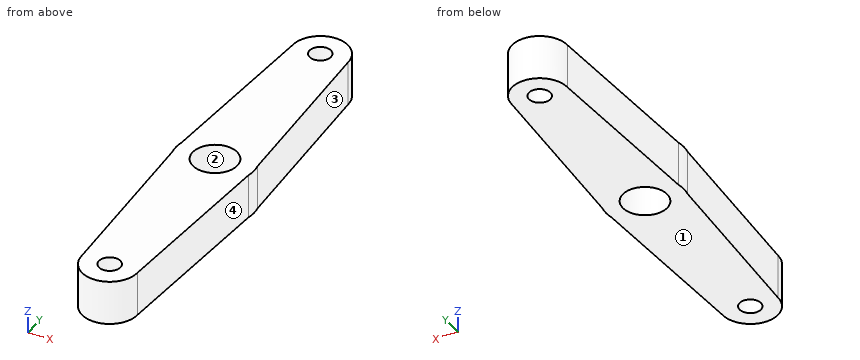
from build123d import *

# Parameters (mm, degrees)
SKETCH001_R   = 2
SKETCH001_R_2 = 0.965047
PAD_DEPTH     = 4


with BuildPart() as part:
    # Sketch001 → Pad (new body)
    with BuildSketch(Plane.XY):
        with BuildLine():
            ThreePointArc((-3.420895, 0.739919), (-3.5, 0), (-3.420895, -0.739919))
            Line((-2.5, -17), (-3.420895, -0.739919))
            ThreePointArc((-2.5, -17), (0, -19.5), (2.5, -17))
            Line((2.5, -17), (3.420895, -0.739919))
            ThreePointArc((3.420895, -0.739919), (3.5, 0), (3.420895, 0.739919))
            Line((3.420895, 0.739919), (2.5, 17))
            ThreePointArc((2.5, 17), (0, 19.5), (-2.5, 17))
            Line((-3.420895, 0.739919), (-2.5, 17))
        make_face()
        Circle(SKETCH001_R, mode=Mode.SUBTRACT)
        with Locations((0, 17)):
            Circle(SKETCH001_R_2, mode=Mode.SUBTRACT)
        with Locations((0, -17)):
            Circle(SKETCH001_R_2, mode=Mode.SUBTRACT)
    extrude(amount=PAD_DEPTH)


solid = part.part
Geometry: final body of the model. Coordinates: model frame, mm. Face numbers are marked on the shaded views. Give positions to 0.01 mm unless a question says otherwise; leave off trailing zeros. Loops run counter-clockwise (first coordinate to the right, second up) from the corner with the lowest first, then second, coordinate; pieces in that order, holes last. Notation, with made-up numbers: M 85,74 L 107,74 A22 ccw 107,106 Z; hole C -11,-20.5 d1. An arc over 180 degrees is marked long. Put each result on its own line as item: value. Start each with the question number.
1) Cut plane A-A (x = 0). Output: boundary loops of the cut face in (y, z).
2) Pull-direction query (Y, two-part tool) for the marked faces 1, 2, 3 and 4; classes: pulls with the +Y half, pulls with the -Y half, needs draft (parallel to the pull), parting line crosses it, or undercut.
3) Cut plane C-C (z = 2.25). Output: boundary loops of the cut face in (x, y).
4) Ray query, line 1 along Y through (x, z) = (0, 1.2); line 2 along Y through (x, z) = (-0.5, 3.75); line 3 along X through (y, z) = (18.5, 0.4). Return the intervals inside material, ascending.
5) Cut plane D-D (y = 10.5). Output: boundary loops of the cut face in (x, z).
6) Cut plane B-B (y = -1.5). Output: boundary loops of the cut face in (x, z), then the cut area to 3 significant figures.
7) Contact query for a flat-ended pin moving along its axis: pin 1 (1.7 mm diameter, centred on x = 0, y = 17, fed in from -Z). Output: stop coordinate, or through.
Verdict:
1. outline: M -19.5,0 L -17.97,0 L -17.97,4 L -19.5,4 Z; M -16.03,0 L -2,0 L -2,4 L -16.03,4 Z; M 2,0 L 16.03,0 L 16.03,4 L 2,4 Z; M 17.97,0 L 19.5,0 L 19.5,4 L 17.97,4 Z
2. face 1: needs draft
2. face 2: undercut
2. face 3: pulls with the +Y half
2. face 4: pulls with the -Y half
3. outline: M -3.42,-0.74 L -2.5,-17 A2.5 ccw 2.5,-17 L 3.42,-0.74 A3.5 ccw 3.42,0.74 L 2.5,17 A2.5 ccw -2.5,17 L -3.42,0.74 A3.5 ccw Z; hole C 0,0 d4; hole C 0,-17 d1.93; hole C 0,17 d1.93
4. line 1: -19.5 to -17.97, -16.03 to -2, 2 to 16.03, 17.97 to 19.5
4. line 2: -19.45 to -17.83, -16.17 to -1.94, 1.94 to 16.17, 17.83 to 19.45
4. line 3: -2 to 2
5. outline: M -2.87,0 L 2.87,0 L 2.87,4 L -2.87,4 Z
6. outline: M -3.38,0 L -1.32,0 L -1.32,4 L -3.38,4 Z; M 1.32,0 L 3.38,0 L 3.38,4 L 1.32,4 Z
6. area: 16.4 mm2
7. pin 1: through
